```python
from build123d import *

# Parameters (mm, degrees)
SKETCH1_R           = 1.375
BOSS_EXTRUDE1_DEPTH = 4


with BuildPart() as part:
    # Sketch1 → Boss-Extrude1 (new body)
    with BuildSketch(Plane(origin=(0, 0, 0), x_dir=(1, 0, 0), z_dir=(0, 1, 0))):
        with BuildLine():
            Line((55, 0), (280, 0))
            ThreePointArc((280, 0), (318.890872965, 16.109127035), (335, 55))
            Line((335, 55), (335, 71))
            Line((335, 71), (313.5, 71))
            Line((313.5, 71), (313.5, 75.5))
            ThreePointArc((313.5, 75.5), (310.5, 78.5), (307.5, 75.5))
            Line((307.5, 75.5), (307.5, 71))
            Line((307.5, 71), (255.5, 71))
            Line((255.5, 71), (255.5, 75.5))
            ThreePointArc((255.5, 75.5), (254.621320344, 77.621320344), (252.5, 78.5))
            Line((252.5, 78.5), (248, 78.5))
            Line((248, 78.5), (248, 121.5))
            Line((248, 121.5), (252.5, 121.5))
            ThreePointArc((252.5, 121.5), (254.621320344, 122.378679656), (255.5, 124.5))
            Line((255.5, 124.5), (255.5, 129))
            Line((255.5, 129), (307.5, 129))
            Line((307.5, 129), (307.5, 124.5))
            ThreePointArc((307.5, 124.5), (310.5, 121.5), (313.5, 124.5))
            Line((313.5, 124.5), (313.5, 129))
            Line((313.5, 129), (335, 129))
            Line((335, 129), (335, 145))
            ThreePointArc((335, 145), (318.890872965, 183.890872965), (280, 200))
            Line((280, 200), (55, 200))
            ThreePointArc((55, 200), (16.109127035, 183.890872965), (0, 145))
            Line((0, 145), (0, 55))
            ThreePointArc((0, 55), (16.109127035, 16.109127035), (55, 0))
        make_face()
        with Locations(Location((252.5, 124.5, 0), (0, 0, 270))):
            Circle(SKETCH1_R, mode=Mode.SUBTRACT)
        with Locations(Location((252.5, 75.5, 0), (0, 0, 90))):
            Circle(SKETCH1_R, mode=Mode.SUBTRACT)
        with Locations(Location((310.5, 124.5, 0), (0, 0, 270))):
            Circle(SKETCH1_R, mode=Mode.SUBTRACT)
        with Locations(Location((310.5, 75.5, 0), (0, 0, 90))):
            Circle(SKETCH1_R, mode=Mode.SUBTRACT)
        with BuildLine():
            Line((55, 25), (280, 25))
            ThreePointArc((280, 25), (297.748239349, 30.813226755), (308.618176043, 46))
            Line((308.618176043, 46), (223, 46))
            Line((223, 46), (223, 154))
            Line((223, 154), (308.618176043, 154))
            ThreePointArc((308.618176043, 154), (297.748239349, 169.186773245), (280, 175))
            Line((280, 175), (55, 175))
            ThreePointArc((55, 175), (33.786796564, 166.213203436), (25, 145))
            Line((25, 145), (25, 55))
            ThreePointArc((25, 55), (33.786796564, 33.786796564), (55, 25))
        make_face(mode=Mode.SUBTRACT)
    extrude(amount=BOSS_EXTRUDE1_DEPTH)


solid = part.part
```
CAD build for the part. Positions are in the model's coordinates, mm. A direction names the side the tool comes from. Give positions to 0.01 mm unless a question says otherwise; leave off trailing zeros. Order: outer loops, then holes, each group sorted by start corner. A loop starts at its lowest first (then second) coordinate and runs counter-clockwise, first axis right, second up.
(1) Saw through at B-B, the plane x = 128.5. Give the cut face in (y, z).
(2) Drill centre lines: L1, parallel to X at y = 2.7, z = -124.5 (3 decimals); L2, parallel to Z at x = 275.5, y = 0.4; L3, parallel to Z at x = 252.5, y = 2.6 (3 decimals). Where is each one in solid material? Low to high.
(3) Saw through at C-C, the plane z = -33.5. Give the cut face in (x, y).
(4) Saw through at D-D, the plane y = 1.7. State how many separate pieces and enclosed holes the cut face has, then the cut area to 3 significant figures.
(5) Flat gauge pins, fed straight in: pin 1 (3 mm diameter, centred on x = 252.5, z = -124.5, fed in from -Y); pin 2 (2 mm diameter, centred on x = 288.5, y = 1.5, fed in from +Z); pin 3 (2 mm diameter, centred on x = 291, y = 3, fed in from -Z); pin 4 (2 mm diameter, centred on y = 1.5, z = -126.5, fed in from +X). Where does each tip first touch, or does it go through?
(6) Mould opens along Z. For faces 1 (the cylindrical face through (15.684, 1.972, -16.539)), 2 (the cylindrical face through (319.316, 1.972, -183.461)), 3 (the cylindrical face through (298, 2, -169)), 4 (the flat face through (240, 0, -101)) say: released by +Z, released by -Z, zero draft, split by the parting line, or undercut.
(7) Saw through at A-A, the plane x = 266. Give the cut face in (y, z), then the cut area to 3 significant figures.
(8) Tool access for faces 5 (the cylindrical face through (34.021, 1.972, -166.445)), 6 (the cylindrical face through (16.539, 1.972, -184.316)): list every direction of +Z, -Z, +X, -X, +Y, -Y with a clear straight run to the whole face (end or side of a thin tool).
Results found:
1. outline: (0, -200) - (4, -200) - (4, -175) - (0, -175) - close; (0, -25) - (4, -25) - (4, 0) - (0, 0) - close
2. L1: x = 0 to 25, 223 to 251.125, 253.875 to 255.5, 307.5 to 309.125, 311.875 to 313.5
2. L2: z = -200 to -175, -154 to -129, -71 to -46, -25 to 0
2. L3: z = -200 to -175, -154 to -125.875, -123.125 to -121.5, -78.5 to -76.875, -74.125 to -46, -25 to 0
3. outline: (4.38, 0) - (34.08, 0) - (34.08, 4) - (4.38, 4) - close; (300.92, 0) - (330.62, 0) - (330.62, 4) - (300.92, 4) - close
4. separate pieces: 1
4. enclosed holes: 5
4. area: 26,900 mm2
5. pin 1: stops at y = 0
5. pin 2: stops at z = -0.51
5. pin 3: stops at z = -199.08
5. pin 4: stops at x = 313.5
6. face 1: released by +Z
6. face 2: released by -Z
6. face 3: undercut
6. face 4: zero draft
7. outline: (0, -200) - (4, -200) - (4, -175) - (0, -175) - close; (0, -154) - (4, -154) - (4, -129) - (0, -129) - close; (0, -71) - (4, -71) - (4, -46) - (0, -46) - close; (0, -25) - (4, -25) - (4, 0) - (0, 0) - close
7. area: 400 mm2
8. face 5: +Y, -Y
8. face 6: -Z, -X, +Y, -Y
